Check sheet for the drawn part. Datum: minimum x, y, z corner. Units: mm. A direction names the side the tool comes from. Round coordinates to 2 decimals unless told otherwise and drop trailing zeros. Order: outer loops, then holes, each group sorted by start corner. A loop starts at its lowest first (then second) coordinate and runs counter-clockwise, first axis right, second up. Notation, with made-up numbers: M 29.25,44 L 69.25,44 A24 cw 69.25,54 Z; hole C -32.5,19 d4. An arc over 180 degrees is marked long. Use one line per item in the form item = value. Start each with the question number.
Item 1: Go/stop test with flat-tipped pins: pin 1 Ø5 at (x, y) = (13.5, 26) entering from +Z; pin 2 Ø4 at (y, z) = (14, 14.5) entering from +X; pin 3 Ø6 at (y, z) = (33.5, 10.5) entering from +X; pin 4 Ø4 at (x, y) = (39.5, 22) entering from +Z. Record where each tip stops, or that it passes through.
Item 2: Cross-section at C-C on y = 20.5. Enter the section's corners in (x, z).
Item 3: Cross-section at B-B on x = 13.25. Enter the section's corners in (y, z) (1 decimal).
Item 4: Thickness scan on probe 1 along Y at (x, z) = (13.25, 38.4) (1 decimal); probe 2 along Y at (x, z) = (39.5, 39.3) (1 decimal); probe 3 along Z at (x, y) = (7, 7.5). Record the ranges inside material, lowest first. Write a range as [from, to].
Item 5: Cross-section at A-A on x = 39.5. Enter the section's corners in (y, z).
Item 6: Tool access check on the marked faces 1, 2 and 3. Record the directions out of +Z, -Z, +X, -X, +Y, -Y that give a thin tool (end or side, any length) a straight path to the whole face; none if there is none.
Item 7: Cross-section at D-D on z = 49. Enter the section's corners in (x, y).
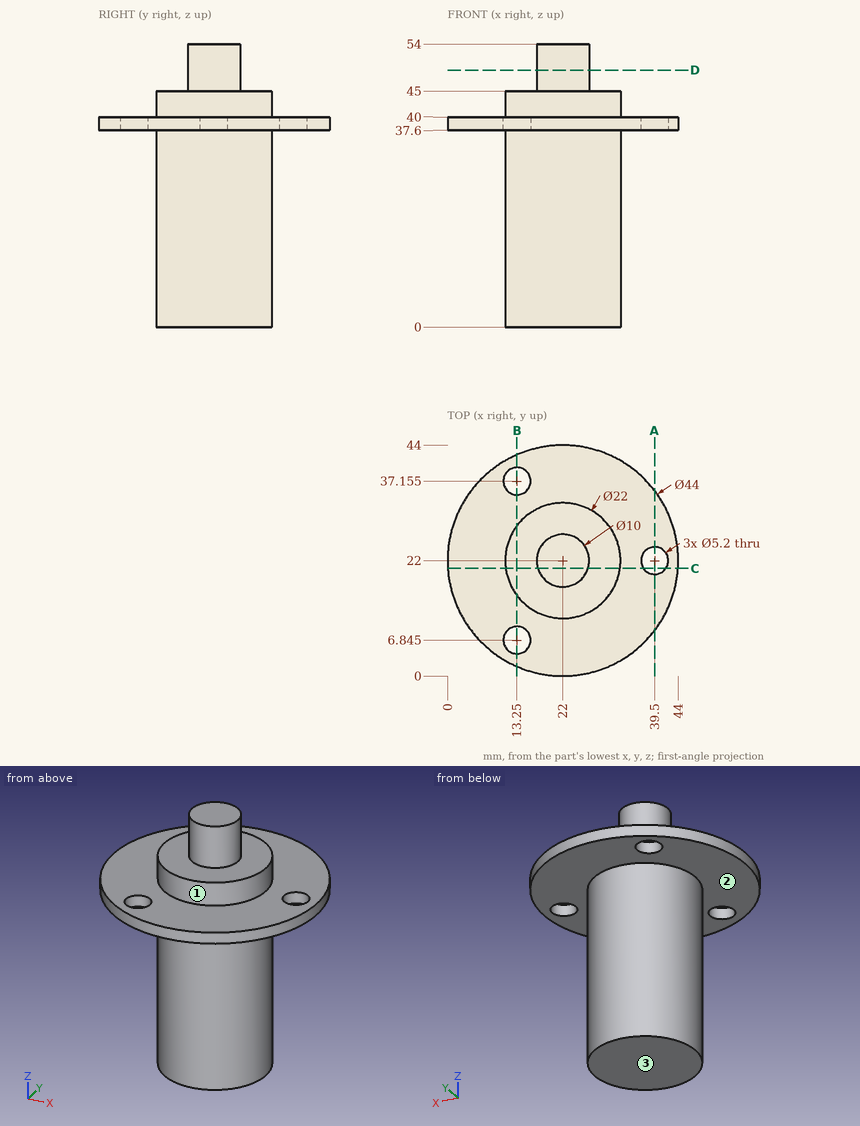
Output values:
q1.pin_1 = 45
q1.pin_2 = 31.22
q1.pin_3 = 28.98
q1.pin_4 = through
q2.outline = M 0.05,37.6 L 11.1,37.6 L 11.1,0 L 32.9,0 L 32.9,37.6 L 37.38,37.6 L 37.38,40 L 32.9,40 L 32.9,45 L 26.77,45 L 26.77,54 L 17.23,54 L 17.23,45 L 11.1,45 L 11.1,40 L 0.05,40 Z; M 41.62,37.6 L 43.95,37.6 L 43.95,40 L 41.62,40 Z
q3.outline = M 1.8,37.6 L 4.2,37.6 L 4.2,40 L 1.8,40 Z; M 9.4,37.6 L 15.3,37.6 L 15.3,0 L 28.7,0 L 28.7,37.6 L 34.6,37.6 L 34.6,40 L 28.7,40 L 28.7,45 L 15.3,45 L 15.3,40 L 9.4,40 Z; M 39.8,37.6 L 42.2,37.6 L 42.2,40 L 39.8,40 Z
q4.probe_1 = [1.8, 4.2], [9.4, 34.6], [39.8, 42.2]
q4.probe_2 = [8.7, 19.4], [24.6, 35.3]
q4.probe_3 = [37.6, 40]
q5.outline = M 8.67,37.6 L 19.4,37.6 L 19.4,40 L 8.67,40 Z; M 24.6,37.6 L 35.33,37.6 L 35.33,40 L 24.6,40 Z
q6.face_1 = +Z
q6.face_2 = -Z
q6.face_3 = -Z, +X, -X, +Y, -Y
q7.outline = C 22,22 d10
